Could you check a few things on this drawing? It's one solid part, dimensions in mm from its lowest x, y, z. Round coordinates to 2 decimals unless told otherwise and drop trailing zeros. Loops run counter-clockwise (first coordinate to the right, second up) from the corner with the lowest first, then second, coordinate; pieces in that order, holes last. Notation, with made-up numbers: M -33,12.5 L -29,12.5 A23 ccw -29,28.5 Z; hole C 44,14 d10. An arc over 180 degrees is marked long. Answer as a JSON object with one key per item and string values.
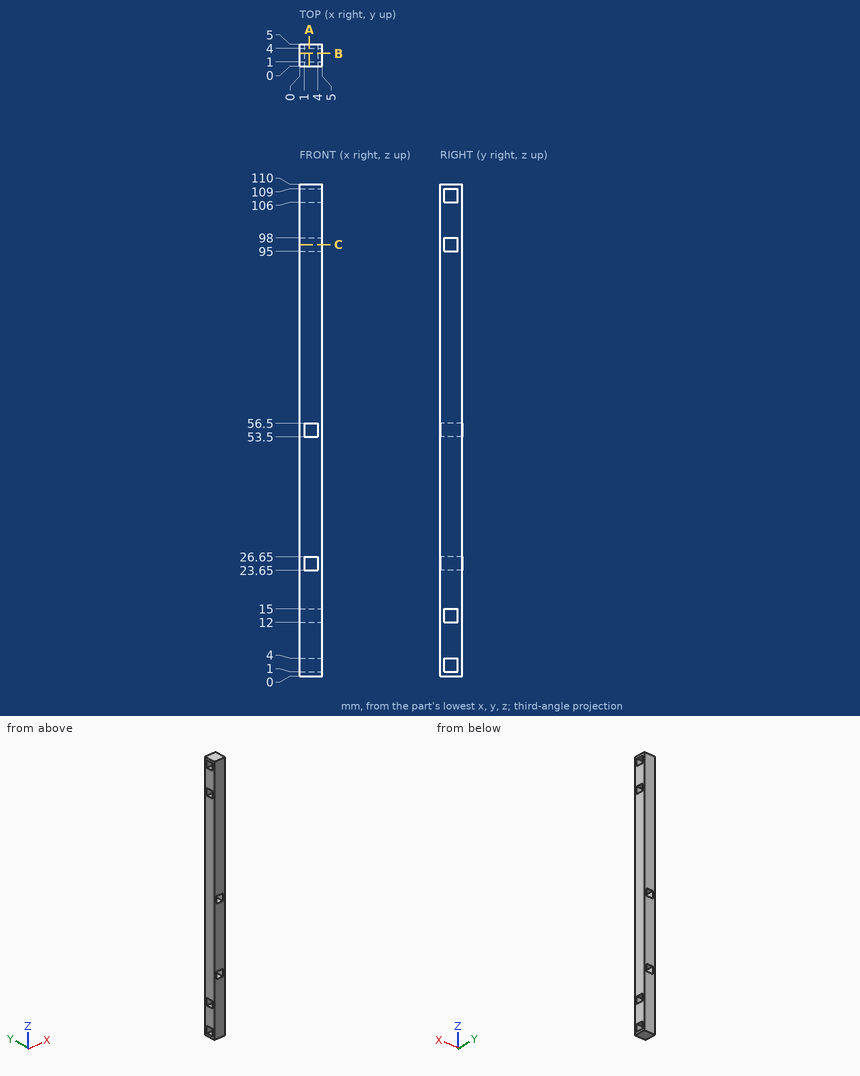
Item 1: I want a section at B-B, the plane y = 2.9. Please give me the cut outline in (x, z).
Resolved:
{"outline": "M 0,0 L 5,0 L 5,1 L 0,1 Z; M 0,4 L 5,4 L 5,12 L 0,12 Z; M 0,15 L 5,15 L 5,95 L 0,95 Z; M 0,98 L 5,98 L 5,106 L 0,106 Z; M 0,109 L 5,109 L 5,110 L 0,110 Z; hole M 1,23.65 L 4,23.65 L 4,26.65 L 1,26.65 Z; hole M 1,53.5 L 4,53.5 L 4,56.5 L 1,56.5 Z"}
Item 2: I want a section at A-A, the plane x = 2.2. Please give me the cut outline in (y, z).
Resolved:
{"outline": "M 0,0 L 5,0 L 5,23.65 L 0,23.65 Z; M 0,26.65 L 5,26.65 L 5,53.5 L 0,53.5 Z; M 0,56.5 L 5,56.5 L 5,110 L 0,110 Z; hole M 1,1 L 4,1 L 4,4 L 1,4 Z; hole M 1,12 L 4,12 L 4,15 L 1,15 Z; hole M 1,95 L 4,95 L 4,98 L 1,98 Z; hole M 1,106 L 4,106 L 4,109 L 1,109 Z"}
Item 3: I want a section at C-C, the plane z = 96.5. Please give me the cut outline in (x, y), then the cut area to 3 significant figures.
Resolved:
{"outline": "M 0,0 L 5,0 L 5,1 L 0,1 Z; M 0,4 L 5,4 L 5,5 L 0,5 Z", "area": "10.0 mm²"}
Item 4: Please list where these lines run through material, in increasing order: probe 1 along Z at (x, y) = (4.85, 3.2); probe 2 along Z at (x, y) = (3.15, 0.2); probe 3 along Y at (x, z) = (2.5, 97). Write a range as from..to.
Resolved:
{"probe 1": "0..1, 4..12, 15..95, 98..106, 109..110", "probe 2": "0..23.65, 26.65..53.5, 56.5..110", "probe 3": "0..1, 4..5"}
